Check sheet for the modelled part. Datum: model origin and axes. Units: mm. Give positions to 0.01 mm unless a question says otherwise; leave off trailing zeros. Write each loop counter-clockwise with the first axis right and the second up, starting at its lowest first coordinate (ties: lowest second). Pieces come first, ordered by that corner, then holes. Notation, with made-up numbers: M -9,29.25 L 14,29.25 A4 cw 14,36.25 Z; hole C 14,-6 d2. An arc over 180 degrees is marked long. Write each question's results on one line, items separated by ' | '. Start each with the question number.
Solid Edge part; units mm, degrees
sketch "Sketch1" plane through (0, 0, 0) normal (0, -1, 0) x (1, 0, 0)
  line L0 (-40, 40) -> (40, 40)
  line L1 (40, 40) -> (40, -40)
  line L2 (40, -40) -> (-40, -40)
  line L3 (-40, -40) -> (-40, 40)
  dimension "D1" = 40
  dimension "D2" = 40
extrude "Protrusion1" add sketch "Sketch1" against normal blind 32
sketch "Sketch2" plane through (40, 16, 0) normal (1, 0, 0) x (0, 1, 0)
  circle A0 centre (0, -40) radius 16
extrude "Cutout1" cut sketch "Sketch2" against normal through all
sketch "Sketch3" plane through (0, 0, 0) normal (0, -1, 0) x (1, 0, 0)
  circle A0 centre (0, 10) radius 15
extrude "Cutout2" cut sketch "Sketch3" against normal through all
Q1. Section check D-D on x = -20.5. Record the boundary of the cut face in (y, z), plus the area to 3 significant figures.
Q2. Section check B-B on x = 0. Record the boundary of the cut face in (y, z).
Q3. Scan lines: L1, parallel to Z at x = 0, y = 16; L2, parallel to X at y = 18.5, z = 13; L3, parallel to Y at x = 9, z = -26. Record each from-to range of solid material in increasing order.
Q4. Section check A-A on z = 10. Record the boundary of the cut face in (x, y).
Q5. Section check C-C on y = 16. Record the boundary of the cut face in (x, z), plus the area to 3 significant figures.
Q6. Release check for a two-part mould opening along Z. For faces 1 (the face through (-1, 16, 40)), 2 (the face through (-1.953, 15.776, 24.872)), 3 (the face through (1, 16, -24)) record: pulls with the +Z half, pulls with the -Z half, needs draft (parallel to the pull), parting line crosses it, or undercut.
Check result:
1) outline: M 0,-40 A16 cw 32,-40 L 32,40 L 0,40 Z | area: 2,160 mm^2
2) outline: M 0,-40 A16 cw 32,-40 L 32,-5 L 0,-5 Z; M 0,25 L 32,25 L 32,40 L 0,40 Z
3) L1: -24 to -5, 25 to 40 | L2: -40 to -14.7, 14.7 to 40 | L3: 0 to 8.25, 23.75 to 32
4) outline: M -40,0 L -15,0 L -15,32 L -40,32 Z; M 15,0 L 40,0 L 40,32 L 15,32 Z
5) outline: M -40,-24 L 40,-24 L 40,40 L -40,40 Z; hole C 0,10 d30 | area: 4,410 mm^2
6) face 1: pulls with the +Z half | face 2: undercut | face 3: pulls with the -Z half
